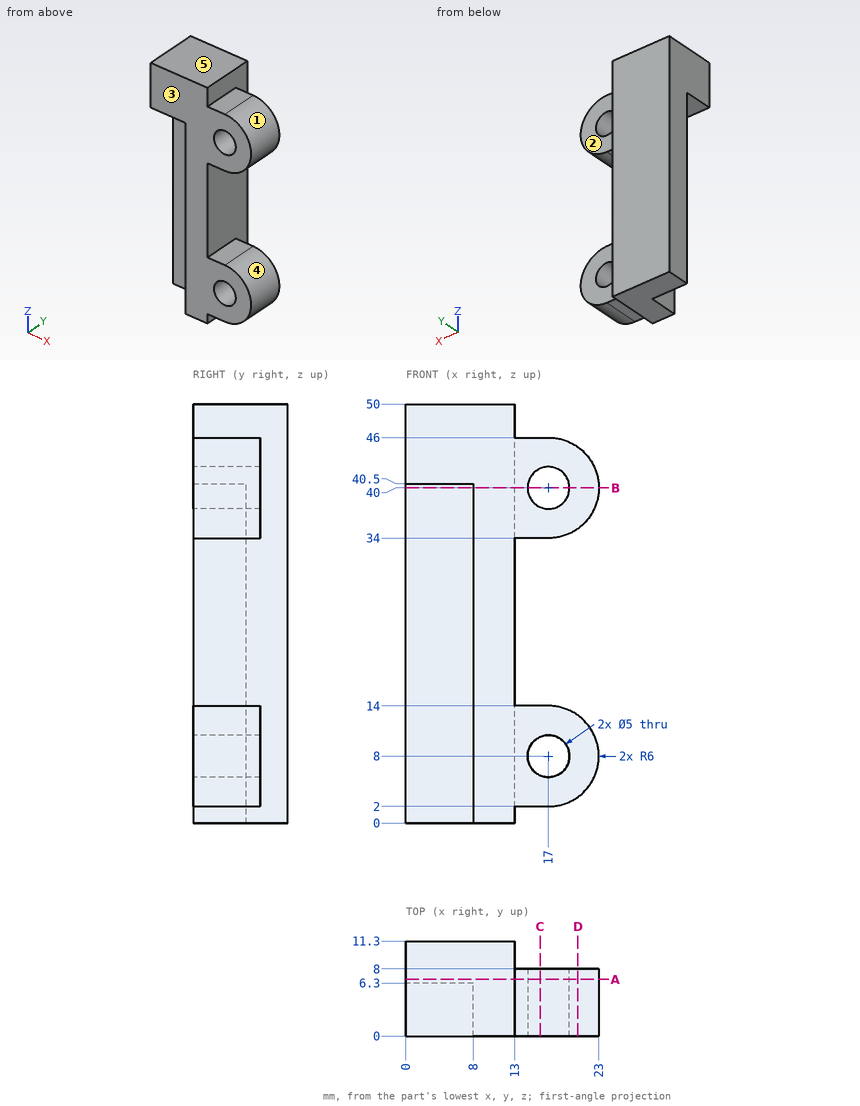
Can you work these out from the drawing? Everything is in mm from the part's minimum corner. A direction names the side the tool comes from. Coordinates: 2 decimals unless noted, no trailing zeros. Loops run counter-clockwise (first coordinate to the right, second up) from the corner with the lowest first, then second, coordinate; pieces in that order, holes last.
1) Imagine slicing it at C-C on x = 16. List the corners of the cut face in (y, z) for me.
2) Imagine slicing it at D-D on x = 20.5. List the corners of the cut face in (y, z) for me, plus the area to 3 significant figures.
3) Thinking about a two-plate mould opening in Z: for the marked faces 3, 4 and 5, which applies, pulls with the +Z half, pulls with the -Z half, needs draft (parallel to the pull), parting line crosses it, or undercut?
4) I need wall thicknesses on probe 1 along Z at (x, y) = (17, 4.5); probe 2 along X at (y, z) = (6, 8); probe 3 along Y at (x, z) = (3.5, 37.5). Which ranges of each line are inside material? Lowest first, please.
5) Imagine slicing it at B-B on z = 40. List the corners of the cut face in (x, y) for me, plus the area to 4 significant figures.
6) Which directions (+Z, -Z, +X, -X, +Y, -Y) give clear straight access to the entire face, cutting with the end or side of a thin tool? Please do the marked faces 1 and 2.
7) For pin 1 (5 mm diameter, centred on x = 16.5, z = 37.5, fed in from +Y); pin 2 (1.2 mm diameter, centred on x = 15, y = 5.5, fed in from +Z); pin 3 (4.5 mm diameter, centred on x = 15.5, y = 4.5, fed in from -Z), each with a flat end and sliding along its axis, tell me the tip position at first contact or that it passes through.
8) Imagine slicing it at A-A on y = 6.75. List the corners of the cut face in (x, z) for me, plus the area to 3 significant figures.
Completed:
1. outline: (0, 2) - (8, 2) - (8, 5.71) - (0, 5.71) - close; (0, 10.29) - (8, 10.29) - (8, 14) - (0, 14) - close; (0, 34) - (8, 34) - (8, 37.71) - (0, 37.71) - close; (0, 42.29) - (8, 42.29) - (8, 46) - (0, 46) - close
2. outline: (0, 3.13) - (8, 3.13) - (8, 12.87) - (0, 12.87) - close; (0, 35.13) - (8, 35.13) - (8, 44.87) - (0, 44.87) - close
2. area: 156 mm2
3. face 3: needs draft
3. face 4: undercut
3. face 5: pulls with the +Z half
4. probe 1: z = 2 to 5.5, 10.5 to 14, 34 to 37.5, 42.5 to 46
4. probe 2: x = 8 to 14.5, 19.5 to 23
4. probe 3: y = 6.3 to 11.3
5. outline: (0, 6.3) - (8, 6.3) - (8, 0) - (14.5, 0) - (14.5, 8) - (13, 8) - (13, 11.3) - (0, 11.3) - close; (19.5, 0) - (23, 0) - (23, 8) - (19.5, 8) - close
5. area: 136.5 mm2
6. face 1: +X, +Y, -Y
6. face 2: +Z, -Z, +X, +Y
7. pin 1: stops at y = 8
7. pin 2: stops at z = 46
7. pin 3: stops at z = 2
8. outline: (0, 0) - (13, 0) - (13, 2) - (17, 2) arc R6 ccw to (17, 14) - (13, 14) - (13, 34) - (17, 34) arc R6 ccw to (17, 46) - (13, 46) - (13, 50) - (0, 50) - close; hole circle Ø5 at (17, 8); hole circle Ø5 at (17, 40)
8. area: 820 mm2
